The model under review builds one solid part; all positions refer to its coordinate system, in mm. A direction names the side the tool comes from. Coordinates: 2 decimals unless noted, no trailing zeros. Loops run counter-clockwise (first coordinate to the right, second up) from the corner with the lowest first, then second, coordinate; pieces in that order, holes last. Notation, with made-up numbers: (84.25, -5) -> (125.25, -5) arc R22 cw to (125.25, 29) -> close; hole circle Ø6 at (53, 16). An arc over 180 degrees is marked (long way). One line per question, with ' | ' between items. Start each with the question number.
from build123d import *

# Parameters (mm, degrees)
F0_W      = 99.28
F0_H      = 99.28
F1_DEPTH  = 5
F2_R      = 9.975
F3_DEPTH  = 50.12
F4_R      = 6.97414
F5_DEPTH  = 45
F6_W      = 10.15
F6_H      = 33.35
F7_DEPTH  = 51.54
F8_W      = 19.84
F8_H      = 17.26
F9_DEPTH  = 30.101
F10_R     = 1.715
F11_DEPTH = 30.101
F12_W     = 99.28
F12_H     = 26.759172
F13_DEPTH = 55.121
F14_W     = 25.082288
F14_H     = 72.520828
F15_DEPTH = 55.121
F16_W     = 74.197712
F16_H     = 22.137212
F17_DEPTH = 55.121
F18_R     = 1.715
F19_DEPTH = 30.101
F20_W     = 4.45
F20_H     = 0.8
F21_DEPTH = 55.121
F22_R     = 1.72
F23_DEPTH = 55.121
F24_W     = 52.245434
F24_H     = 58.427127
F25_DEPTH = 74.198713


with BuildPart() as f1:
    # F0 (on Top) → F1 (new body)
    with BuildSketch(Plane.XY):
        with Locations((1.248532, -12.53785)):
            Rectangle(F0_W, F0_H)
    extrude(amount=F1_DEPTH)

    # F2 (on face) → F3 (join)
    with BuildSketch(Plane(origin=(0, 0, 0), x_dir=(1, 0, 0), z_dir=(0, 0, -1))):
        with Locations((0, 12.20285)):
            Circle(F2_R)
    extrude(amount=F3_DEPTH)

    # F4 (on face) → F5 (cut)
    with BuildSketch(Plane(origin=(0, 0, -50.12), x_dir=(1, 0, 0), z_dir=(0, 0, -1))):
        with Locations((0, 12.20285)):
            Circle(F4_R)
    extrude(amount=-F5_DEPTH, mode=Mode.SUBTRACT)

    # F6 (on face) → F7 (join)
    with BuildSketch(Plane.XY.offset(5)):
        with Locations((-23.366468, -12.46285)):
            Rectangle(F6_W, F6_H)
    extrude(amount=F7_DEPTH)

    # F8 (on face) → F9 (cut, through all)
    with BuildSketch(Plane.YZ.offset(-18.291468)):
        with Locations((-12.51785, 47.91)):
            Rectangle(F8_W, F8_H)
    extrude(amount=-F9_DEPTH, mode=Mode.SUBTRACT)

    # F10 (on face) → F11 (cut, through all)
    with BuildSketch(Plane.YZ.offset(-18.291468)):
        with Locations((-25.66285, 52.125)):
            Circle(F10_R)
        with Locations((-25.66285, 47.205)):
            Circle(F10_R)
    extrude(amount=-F11_DEPTH, mode=Mode.SUBTRACT)

    # F12 (on face) → F13 (cut, through all)
    with BuildSketch(Plane.XY.offset(5)):
        with Locations((1.248532, 23.722564)):
            Rectangle(F12_W, F12_H)
    extrude(amount=-F13_DEPTH, mode=Mode.SUBTRACT)

    # F14 (on face) → F15 (cut, through all)
    with BuildSketch(Plane.XY.offset(5)):
        with Locations((38.347388, -25.917436)):
            Rectangle(F14_W, F14_H)
    extrude(amount=-F15_DEPTH, mode=Mode.SUBTRACT)

    # F16 (on face) → F17 (cut, through all)
    with BuildSketch(Plane.XY.offset(5)):
        with Locations((-11.292612, -51.109244)):
            Rectangle(F16_W, F16_H)
    extrude(amount=-F17_DEPTH, mode=Mode.SUBTRACT)

    # F18 (on face) → F19 (cut, through all)
    with BuildSketch(Plane.YZ.offset(-18.291468)):
        with Locations((0.73715, 52.125)):
            Circle(F18_R)
        with Locations((0.73715, 47.205)):
            Circle(F18_R)
    extrude(amount=-F19_DEPTH, mode=Mode.SUBTRACT)

    # F20 (on face) → F21 (cut, through all)
    with BuildSketch(Plane.XY.offset(5)):
        with Locations((-16.306812, -38.074275)):
            Rectangle(F20_W, F20_H)
        with Locations((-16.306812, 6.925725)):
            Rectangle(F20_W, F20_H)
        with Locations((9.693188, -38.074275)):
            Rectangle(F20_W, F20_H)
        with Locations((9.693188, 6.925725)):
            Rectangle(F20_W, F20_H)
    extrude(amount=-F21_DEPTH, mode=Mode.SUBTRACT)

    # F22 (on face) → F23 (cut, through all)
    with BuildSketch(Plane.XY.offset(5)):
        with Locations((-43.671468, 5.622978)):
            Circle(F22_R)
        with Locations((-43.671468, -35.377022)):
            Circle(F22_R)
        with Locations((21.328532, 5.622978)):
            Circle(F22_R)
        with Locations((21.328532, -35.377022)):
            Circle(F22_R)
    extrude(amount=-F23_DEPTH, mode=Mode.SUBTRACT)

    # F24 (on face) → F25 (cut, through all)
    with BuildSketch(Plane.YZ.offset(25.806244)):
        with Locations((-13.917921, 31.713563)):
            Rectangle(F24_W, F24_H)
    extrude(amount=-F25_DEPTH, mode=Mode.SUBTRACT)


solid = f1.part
1) Consider section D-D, the plane x = -35. Write out the cut boundary in (y, z), plus the area to 3 significant figures.
2) Wall thickness on L1, parallel to Y at x = 0, z = -35; L2, parallel to Z at x = 12, y = -22.5; L3, parallel to X at y = -11, z = -31: over which ranges is each line inside the solid? List them lowest first.
3) Consider section A-A, the plane x = 0. Write out the cut boundary in (y, z).
4) Consider section C-C, the plane z = -33. Write out the cut boundary in (x, y) (3 decimals), plus the area to 3 significant figures.
5) Consider section B-B, the plane y = -7. Write out the cut boundary in (x, z), plus the area to 3 significant figures.
6) Mouldability with a two-part tool opening along X and no side actions: class faces 4 (the face through (-48.391, -15, 1)), 5 (the face through (-11, -15, 2.5)), 6 (the face through (10, 7.326, 1)) as +X half, -X half, draft (parallel to the pull), parting line (faces both ways), or undercut.
7) Machinability: for faces 1 (the face through (-1.299, -22.093, -24.709)), 2 (the face through (-12, -40.041, 1)), 3 (the face through (-16, -38.474, 1)), which of the approach directions +Z, -Z, +X, -X, +Y, -Y give a long, thin tool a straight path to every point of the face, cutting with its end or side? Answer none if there is none.
8) Insertion check: pin 1 Ø2 at (y, z) = (-8.5, -32.5) entering from +X; pin 2 Ø4 at (y, z) = (-18, -7) entering from -X; pin 3 Ø2 at (y, z) = (-15, -40) entering from +X. Each pin has a flat end and moves straight along its axis. Give the tip position at first contact, or say it passes through.
Filled sheet:
1) outline: (-40.04, 0) -> (10.34, 0) -> (10.34, 2.5) -> (-40.04, 2.5) -> close | area: 126 mm^2
2) L1: -22.18 to -19.18, -5.23 to -2.23 | L2: 0 to 2.5 | L3: -9.9 to -6.87, 6.87 to 9.9
3) outline: (-40.04, 0) -> (-22.18, 0) -> (-22.18, -50.12) -> (-19.18, -50.12) -> (-19.18, -5.12) -> (-5.23, -5.12) -> (-5.23, -50.12) -> (-2.23, -50.12) -> (-2.23, 0) -> (10.34, 0) -> (10.34, 2.5) -> (-40.04, 2.5) -> close
4) outline: circle Ø19.95 at (0, -12.203); hole circle Ø13.948 at (0, -12.203) | area: 160 mm^2
5) outline: (-48.39, 0) -> (-8.51, 0) -> (-8.51, -50.12) -> (-4.64, -50.12) -> (-4.64, -5.12) -> (4.64, -5.12) -> (4.64, -50.12) -> (8.51, -50.12) -> (8.51, 0) -> (25.81, 0) -> (25.81, 2.5) -> (-48.39, 2.5) -> close | area: 621 mm^2
6) face 4: -X half | face 5: draft | face 6: undercut
7) face 1: -Z | face 2: +Z, -Z, +X, -X, -Y | face 3: +Z, -Z
8) pin 1: x = 9.6 | pin 2: x = -9.22 | pin 3: x = 9.81
